Job drawing, mm, ordinate dimensions from the low corner. One solid piece. A direction names the side the tool comes from. Give positions to 0.01 mm unless a question says otherwise; leave off trailing zeros. Order: outer loops, then holes, each group sorted by start corner. A loop starts at its lowest first (then second) coordinate and runs counter-clockwise, first axis right, second up. Notation, with made-up numbers: (37, -9) - (49, -9) arc R10 ccw to (49, -4) - close; hole circle Ø11 at (-32.75, -7.5). An arc over 180 degrees is marked (long way). Use one line per item in the form item = value. Start each with the question number.
1. Band-saw the part on C-C, the plane z = 14. List the corners of the cut face in (x, y), plus the area to 3 significant figures.
2. Band-saw the part on A-A, the plane x = 4. List the corners of the cut face in (y, z).
3. Pull direction Y, two halves, no side cores. Call the marked faces 3, 4 and 5: +Y half, -Y half, draft (parallel to the pull), parting line (faces both ways), or undercut.
4. Drill centre lines: line 1 (X direction, y = 23.15, z = 1); line 2 (Y direction, x = 4, z = 1.35); line 3 (Y direction, x = 5.75, z = 7). Where is each one in solid material? Low to high.
5. Pin check, flat tips, straight feed: P1, Ø2.5, axis at x = 6, z = 9, coming from the +Y side; P2, Ø4, axis at x = 5, y = 19, coming from the +Z side; P3, Ø4, axis at x = 4, y = 23.15, coming from the +Z side. Stop position of each tip, or through.
6. Band-saw the part on B-B, the plane y = 23.15. List the corners of the cut face in (x, z), plus the area to 3 significant figures.
7. Band-saw the part on D-D, the plane z = 1.5. List the corners of the cut face in (x, y).
8. Tool access for the marked faces 1 and 2: list every direction of +Z, -Z, +X, -X, +Y, -Y with a clear straight run to the whole face (end or side of a thin tool).
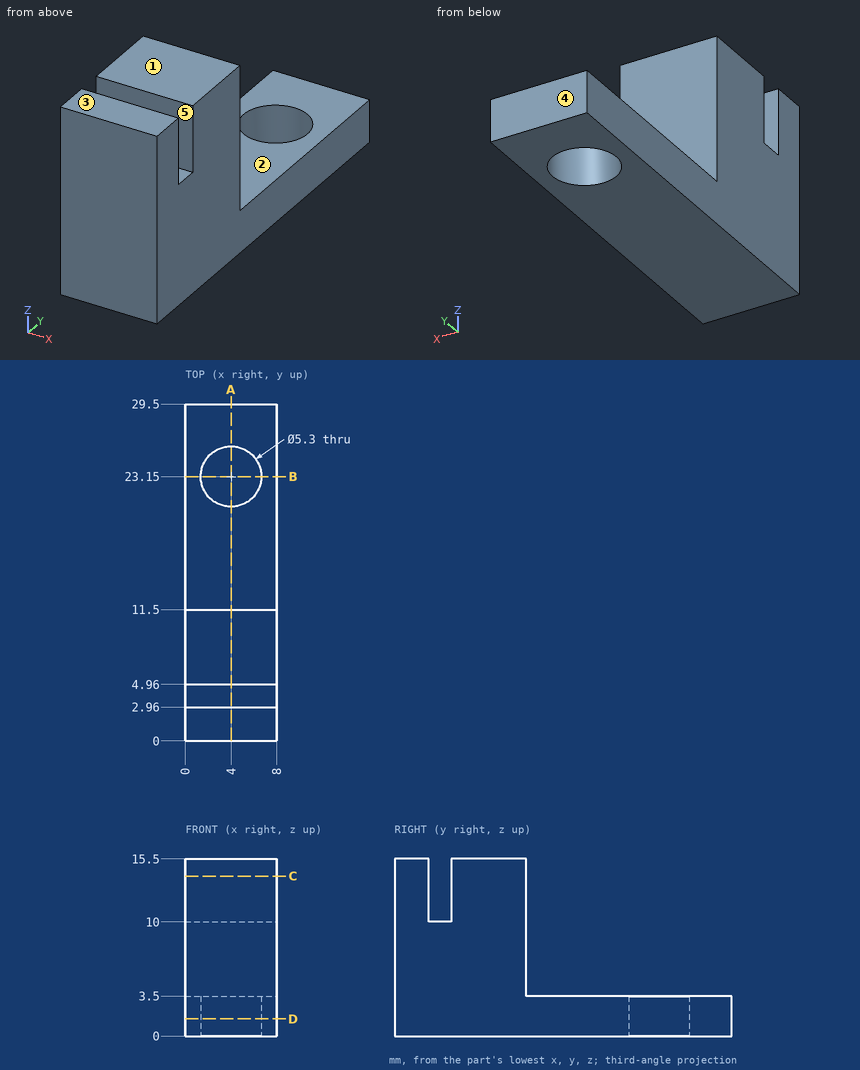
From the geometry:
q1.outline = (0, 0) - (8, 0) - (8, 2.96) - (0, 2.96) - close; (0, 4.96) - (8, 4.96) - (8, 11.5) - (0, 11.5) - close
q1.area = 76.0 mm²
q2.outline = (0, 0) - (20.5, 0) - (20.5, 3.5) - (11.5, 3.5) - (11.5, 15.5) - (4.96, 15.5) - (4.96, 10) - (2.96, 10) - (2.96, 15.5) - (0, 15.5) - close; (25.8, 0) - (29.5, 0) - (29.5, 3.5) - (25.8, 3.5) - close
q3.face_3 = draft
q3.face_4 = +Y half
q3.face_5 = undercut
q4.line_1 = 0 to 1.35, 6.65 to 8
q4.line_2 = 0 to 20.5, 25.8 to 29.5
q4.line_3 = 0 to 11.5
q5.P1 = 11.5
q5.P2 = 3.5
q5.P3 = through
q6.outline = (0, 0) - (1.35, 0) - (1.35, 3.5) - (0, 3.5) - close; (6.65, 0) - (8, 0) - (8, 3.5) - (6.65, 3.5) - close
q6.area = 9.45 mm²
q7.outline = (0, 0) - (8, 0) - (8, 29.5) - (0, 29.5) - close; hole circle Ø5.3 at (4, 23.15)
q8.face_1 = +Z, +X, -X, +Y, -Y
q8.face_2 = +Z, +X, -X, +Y
